Source: CAD feature listing. Evaluate the final solid. Frame: model axes, mm. Face numbers are marked on the shaded views. Coordinates: 2 decimals unless noted, no trailing zeros. Order: outer loops, then holes, each group sorted by start corner. A loop starts at its lowest first (then second) coordinate and runs counter-clockwise, first axis right, second up.
```python
from build123d import *

# Parameters (mm, degrees)
BOSS_EXTRUDE1_DEPTH = 45
FILLET1_R           = 0.4
SKETCH3_R           = 1.5
CUT_EXTRUDE3_DEPTH  = 5
CUT_EXTRUDE5_DEPTH  = 6


with BuildPart() as part:
    # Sketch2 → Boss-Extrude1 (new body)
    with BuildSketch(Plane(origin=(0, 0, 0), x_dir=(1, 0, 0), z_dir=(0, 1, 0))):
        Polygon((-13.5, 5), (13.5, 5), (13.5, -5), (6, -5), (6, -3.75), (5.25, -3), (4, -3), (4, -2), (5.25, -2), (6, -1.25), (6, 0), (-6, 0), (-6, -1.25), (-5.25, -2), (-4, -2), (-4, -3), (-5.25, -3), (-6, -3.75), (-6, -5), (-13.5, -5), align=None)
    extrude(amount=BOSS_EXTRUDE1_DEPTH)

    # Fillet1
    fillet1_edges = [part.edges().sort_by_distance(p)[0] for p in [
        (6, 22.5, 5),
        (-6, 22.5, 5),
    ]]
    fillet(fillet1_edges, radius=FILLET1_R)

    # Sketch3 → Cut-Extrude3 (cut)
    with BuildSketch(Plane(origin=(0, 0, -5), x_dir=(-1, 0, 0), z_dir=(0, 0, -1))):
        with Locations((10, 33.5)):
            Circle(SKETCH3_R)
        with Locations((-10, 33.5)):
            Circle(SKETCH3_R)
        with Locations((-10, 13.5)):
            Circle(SKETCH3_R)
        with Locations((10, 13.5)):
            Circle(SKETCH3_R)
    extrude(amount=-CUT_EXTRUDE3_DEPTH, mode=Mode.SUBTRACT)

    # Sketch4 → Cut-Extrude5 (cut)
    with BuildSketch(Plane(origin=(0, 45, 0), x_dir=(1, 0, 0), z_dir=(0, 1, 0))):
        Polygon((-13.5, 5), (-13.5, 4.25), (-12.75, 5), align=None)
        Polygon((13.5, 4.25), (12.75, 5), (13.5, 5), align=None)
        Polygon((-13.5, -5), (-13.2, -5), (-13.5, -4.7), align=None)
        Polygon((13.2, -5), (13.5, -4.7), (13.5, -5), align=None)
    cut_extrude5 = extrude(amount=-CUT_EXTRUDE5_DEPTH, mode=Mode.SUBTRACT)

    # Mirror1: Cut-Extrude5 across plane
    add(cut_extrude5.mirror(Plane.ZX.offset(21.5)), mode=Mode.SUBTRACT)


solid = part.part
```
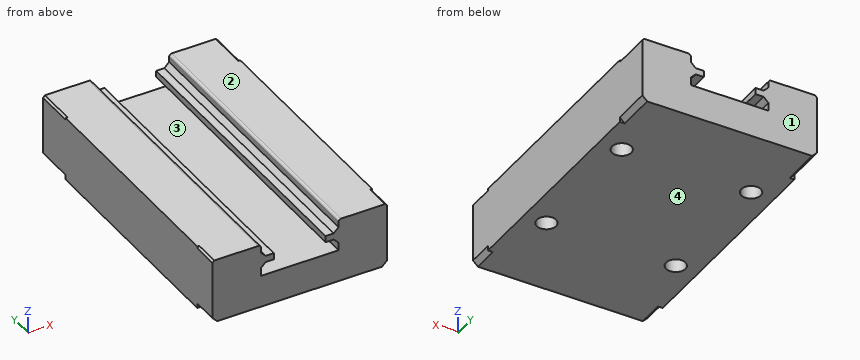
Q1. Pin query (flat end, axial travel): P1, Ø0.6, axis at x = -5, y = 14, coming from the +Z side; P2, Ø1, axis at x = 2.5, z = 3, coming from the -Y side; P3, Ø1.5, axis at x = -9.5, y = 33, coming from the -Z side; P4, Ø3.5, axis at x = -1, y = 27, coming from the +Z side. Return the tip coordinate at first contact, or that it passes through.
Solutions:
P1: stops at z = 3.05
P2: passes through
P3: stops at z = 0
P4: stops at z = 0
Q2. Section query C-C on z = -0.5. Output: boundary loops of the cut face in (x, y), plus the area to 3 significant figures.
Solutions:
outline: (-13.5, 0) - (13.5, 0) - (13.5, 45) - (-13.5, 45) - close; hole circle Ø3 at (-10, 13.5); hole circle Ø3 at (-10, 33.5); hole circle Ø3 at (10, 13.5); hole circle Ø3 at (10, 33.5)
area: 1,190 mm2
Q3. Section query D-D on x = -10. Output: boundary loops of the cut face in (y, z).
Solutions:
outline: (0, -5) - (12, -5) - (12, 0) - (15, 0) - (15, -5) - (32, -5) - (32, 0) - (35, 0) - (35, -5) - (45, -5) - (45, 5) - (0, 5) - close
Q4. Section query A-A on z = 2.5. Output: boundary loops of the cut face in (x, y).
Solutions:
outline: (-13.5, 0) - (-4, 0) - (-4, 45) - (-13.5, 45) - close; (4, 0) - (13.5, 0) - (13.5, 45) - (4, 45) - close
Q5. Section query B-B on y = 21.5. Output: boundary loops of the cut face in (x, z).
Solutions:
outline: (-13.5, -5) - (13.5, -5) - (13.5, 5) - (6.4, 5) arc R0.4 ccw to (6, 4.6) - (6, 3.75) - (5.25, 3) - (4, 3) - (4, 2) - (5.25, 2) - (6, 1.25) - (6, 0) - (-6, 0) - (-6, 1.25) - (-5.25, 2) - (-4, 2) - (-4, 3) - (-5.25, 3) - (-6, 3.75) - (-6, 4.6) arc R0.4 ccw to (-6.4, 5) - (-13.5, 5) - close
Q6. Material intervals for line 1 along Y through (x, z) = (10, -3.15); line 2 along Z through (x, y) = (4.25, 25); line 3 along X through (y, z) = (40.5, 2.75), sorted ascending.
Solutions:
line 1: y = 0 to 12, 15 to 32, 35 to 45
line 2: z = -5 to 0, 2 to 3
line 3: x = -13.5 to -4, 4 to 13.5
Q7. Pull-direction query (Z, two-part tool) for the marked faces 1, 2, 3 and 4; classes: pulls with the +Z half, pulls with the -Z half, needs draft (parallel to the pull), parting line crosses it, or undercut.
Solutions:
face 1: needs draft
face 2: pulls with the +Z half
face 3: undercut
face 4: pulls with the -Z half
